Part model, mm, in its own coordinate system. A direction names the side the tool comes from. Coordinates: 2 decimals unless noted, no trailing zeros. Write each loop counter-clockwise with the first axis right and the second up, starting at its lowest first coordinate (ties: lowest second). Pieces come first, ordered by that corner, then holes. Notation, with made-up numbers: (-24.75, 50) - (-10.75, 50) arc R15 ccw to (-10.75, 72) - close; hole circle Ø6 at (87.25, -34.75). An arc over 180 degrees is marked (long way). Use a Markdown table: item, result.
Autodesk Inventor part; units mm, degrees
ref_plane "YZ Plane" through (0, 0, 0) normal (1, 0, 0) x (0, 1, 0)
ref_plane "XZ Plane" through (0, 0, 0) normal (0, 1, 0) x (-1, 0, 0)
ref_plane "XY Plane" through (0, 0, 0) normal (0, 0, 1) x (1, 0, 0)
sketch "草图1" plane through (0, 0, 0) normal (0, 1, 0) x (-1, 0, 0)
  arc A0 (0, -13) -> (0, 13) centre (0, 0) ccw
  line L0 (0, 0) -> (-30, 0)
  line L1 (0, -13) -> (-30, -5)
  line L2 (-30, 5) -> (0, 13)
  line L3 (-30, 5) -> (-63, 5)
  line L4 (-63, -5) -> (-30, -5)
  arc A1 (-63, 5) -> (-63, -5) centre (-63, 0) ccw
  dimension "d0" = 26
  dimension "d10" = 10
extrude "拉伸1" add sketch "草图1" along normal blind 4
sketch "草图2" plane through (0, 0, 0) normal (0, -1, 0) x (1, 0, 0)
  line L0 (30, 5) -> (63, 5)
  line L1 (0, 13) -> (30, 5)
  arc A0 (0, 13) -> (0, -13) centre (0, 0) ccw
  line L2 (30, -5) -> (0, -13)
  line L3 (63, -5) -> (30, -5)
  circle A1 centre (0, 0) radius 15
  arc A2 (63, -5) -> (63, 5) centre (63, 0) ccw
  dimension "d7" = 30
extrude "拉伸2" add sketch "草图2" along normal blind 4 contours A1 L2 A0 L1 | L1 A0 L2 A1
sketch "草图3" plane through (0, 4, 0) normal (0, 1, 0) x (1, 0, 0)
  line L0 (0, -13) -> (30, -5)
  line L1 (30, -5) -> (63, -5)
  arc A0 (63, -5) -> (63, 5) centre (63, 0) ccw
  line L2 (63, 5) -> (30, 5)
  line L3 (30, 5) -> (0, 13)
  arc A1 (0, 13) -> (0, -13) centre (0, 0) ccw
  line L4 (0, -13) -> (30, -5)
  line L5 (30, -5) -> (0, -5)
  line L6 (0, -5) -> (0, 5)
  line L7 (0, 5) -> (30, 5)
extrude "拉伸3" add sketch "草图3" along normal blind 5 contours L5 L6 L7 L2 A0 L1
sketch "草图4" plane through (0, 0, 0) normal (0, 0, 1) x (1, 0, 0)
  line L0 (0, 0) -> (0, 0)
  line L1 (0, 0) -> (0, 4)
  line L2 (0, 4) -> (0, 4)
  line L3 (0, 0) -> (0, 4)
  line L4 (-15, -4) -> (15, -4)
  line L5 (11.1585, 0) -> (11.1585, 0)
  line L6 (11.1585, 0) -> (11.1585, 0)
  line L7 (0, 4) -> (-13, 4)
  line L8 (-13, 4) -> (-13, 0)
  line L9 (-15, 0) -> (11.1585, 0)
  line L10 (-12, 4) -> (-8, 13)
  line L11 (-8, 13) -> (0, 13)
  line L12 (30, 4) -> (0, 4)
  line L13 (0, 13) -> (0, 4)
  dimension "d14" = 1
  dimension "d15" = 9
  dimension "d16" = 8
revolve "旋转1" add sketch "草图4" angle 360 about axis through (0, 13, 0) along (0, -1, 0) contours L7 L10 L11 L13
sketch "草图5" plane through (0, 13, 0) normal (0, 1, 0) x (1, 0, 0)
  arc A0 (0, -5) -> (0, 5) centre (0, 0) ccw
  line L0 (0, -5) -> (-5, 0)
  line L1 (-5, 0) -> (0, 5)
  dimension "d18" = 10
extrude "拉伸4" cut sketch "草图5" against normal through all
properties part number "4-手柄" material "灰口铁"
Item 1: Band-saw the part on A-A, the plane y = 2.75. Give the cut face in (x, z).
From the geometry:
| item | result |
|---|---|
| outline | (0, -13) - (30, -5) - (63, -5) arc R5 ccw to (63, 5) - (30, 5) - (0, 13) arc R13 ccw to start; hole (-5, 0) - (0, -5) arc R5 ccw to (0, 5) - close |
Item 2: Drill centre lines: probe 1 along Z at (x, y) = (44, 5.5); probe 2 along Y at (x, z) = (7, 12); probe 3 along X at (y, z) = (11.5, 3.75). Where is each one in solid material? Low to high.
From the geometry:
| item | result |
|---|---|
| probe 1 | -5 to 5 |
| probe 2 | -4 to 0 |
| probe 3 | -7.81 to -1.25, 3.31 to 7.81 |
Item 3: Drop flat-ended pins along their axis: P1, Ø4.5, axis at x = 48.5, y = 2.5, coming from the +Z side; P2, Ø1.5, axis at y = 6.5, z = 9.5, coming from the +X side; P3, Ø6, axis at x = 19, z = 1, coming from the +Y side. Give the stop position or say it passes through.
From the geometry:
| item | result |
|---|---|
| P1 | z = 5 |
| P2 | x = 6.63 |
| P3 | y = 9 |
Item 4: Band-saw the part on D-D, the plane x = 40.5. Give the cut face in (y, z).
From the geometry:
| item | result |
|---|---|
| outline | (0, -5) - (9, -5) - (9, 5) - (0, 5) - close |
Item 5: Band-saw the part on C-C, the plane y = 8. Give the cut face in (x, z).
From the geometry:
| item | result |
|---|---|
| outline | (8.92, -5) - (63, -5) arc R5 ccw to (63, 5) - (8.92, 5) arc R10.22 ccw (long way) to start; hole (-5, 0) - (0, -5) arc R5 ccw to (0, 5) - close |
Item 6: Band-saw the part on B-B, the plane x = 29. Give the cut face in (y, z), then the cut area to 3 significant figures.
From the geometry:
| item | result |
|---|---|
| outline | (0, -5.27) - (4, -5.27) - (4, -5) - (9, -5) - (9, 5) - (4, 5) - (4, 5.27) - (0, 5.27) - close |
| area | 92.1 mm^2 |
Item 7: Two-plate mould, pull along X, no slides. Class faces 1 (the face through (5, 5, 0)), 2 (the face through (-13, 0, 3)), 3 (the face through (-14.985, -1.972, -0.66)): pulls with the +X half, pulls with the -X half, needs draft (parallel to the pull), parting line crosses it, or undercut.
From the geometry:
| item | result |
|---|---|
| face 1 | undercut |
| face 2 | needs draft |
| face 3 | parting line crosses it |
Item 8: Which spindle directions (+Z, -Z, +X, -X, +Y, -Y) get a long thin tool onto all of the face, cutting with end or side? Do faces 4 (the face through (41, 5, -5)), 5 (the face through (12, 4, -6)), 6 (the face through (42, 4, 5)). Say none if no direction does.
From the geometry:
| item | result |
|---|---|
| face 4 | -Z, +X, +Y |
| face 5 | +Y |
| face 6 | +Z, +X, +Y |
